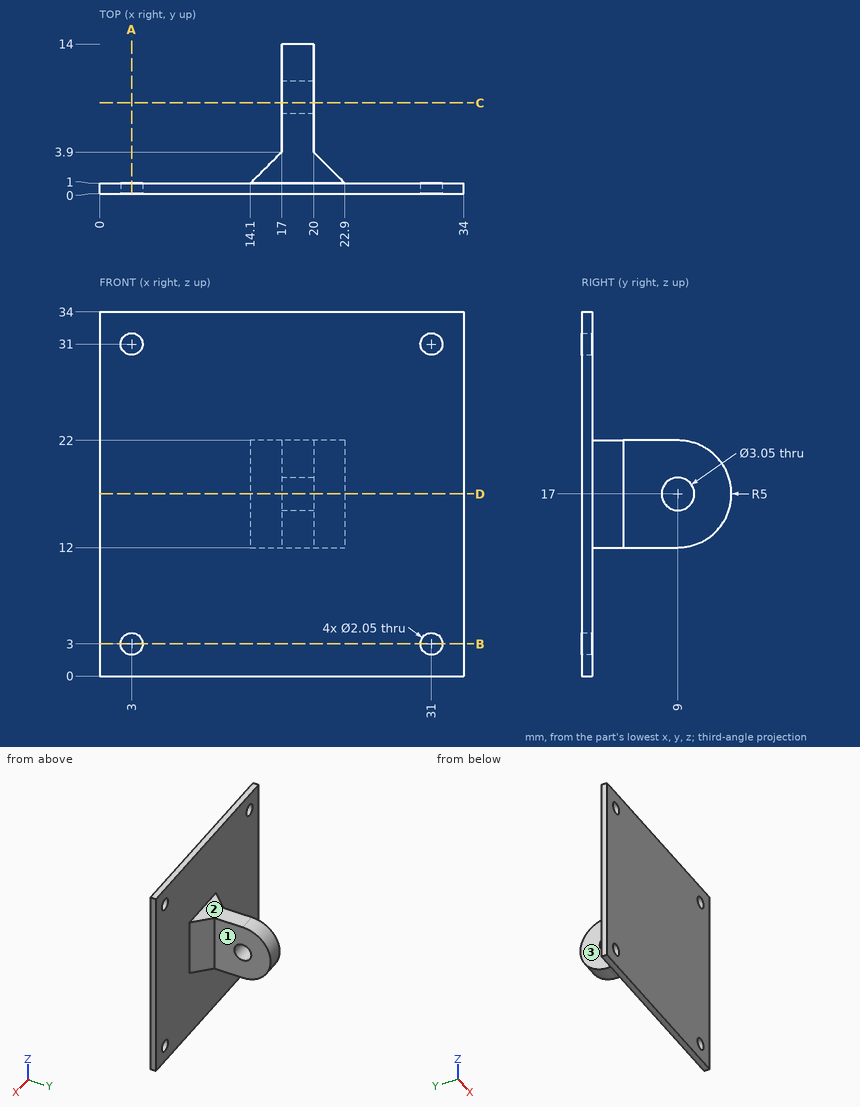
Job drawing, mm, ordinate dimensions from the low corner. One solid piece. A direction names the side the tool comes from. Coordinates: 2 decimals unless noted, no trailing zeros. Order: outer loops, then holes, each group sorted by start corner. A loop starts at its lowest first (then second) coordinate and runs counter-clockwise, first axis right, second up. Notation, with made-up numbers: (-25.5, 58.5) - (-4.5, 58.5) arc R25 cw to (-4.5, 84.5) - close; hole circle Ø5 at (61.5, -8). An arc over 180 degrees is marked (long way). Return JSON: item names as keys, results as strings. Group by question number.
1) Flat gauge pins, fed straight in: P1, Ø4, axis at y = 1.5, z = 19.5, coming from the +X side; P2, Ø2, axis at x = 26.5, z = 5, coming from the +Y side; P3, Ø3, axis at y = 11, z = 16, coming from the +X side; P4, Ø3, axis at y = 10, z = 18.5, coming from the -X side. Where does each tip first touch, or does it go through?
2) Saw through at B-B, the plane z = 3. Write the cut outline in (x, y) (3 decimals).
3) Saw through at D-D, the plane z = 17. Write the cut outline in (x, y) (3 decimals).
4) Saw through at C-C, the plane y = 8.5. Write the cut outline in (x, z), plus the area to 3 significant figures.
5) Probe line 1 (X direction, y = 0.5, z = 3) (3 decimals); line 2 (Y direction, x = 24, z = 10); line 3 (Y direction, x = 18, z = 17) (3 decimals). List the from-to ranges inside material, lowest first. Write a range as from..to.
6) Saw through at A-A, the plane x = 3. Write the cut outline in (y, z) (3 decimals), plus the area to 3 significant figures.
7) Tool access for the marked faces 1, 2 and 3: list every direction of +Z, -Z, +X, -X, +Y, -Y with a clear straight run to the whole face (end or side of a thin tool).
Values found:
{
 "1": {"P1": "stops at x = 34", "P2": "stops at y = 1", "P3": "stops at x = 20", "P4": "stops at x = 17"},
 "2": {"outline": "(0, 0) - (1.975, 0) - (1.975, 1) - (0, 1) - close; (4.025, 0) - (29.975, 0) - (29.975, 1) - (4.025, 1) - close; (32.025, 0) - (34, 0) - (34, 1) - (32.025, 1) - close"},
 "3": {"outline": "(0, 0) - (34, 0) - (34, 1) - (22.9, 1) - (20, 3.9) - (20, 7.475) - (17, 7.475) - (17, 3.9) - (14.1, 1) - (0, 1) - close; (17, 10.525) - (20, 10.525) - (20, 14) - (17, 14) - close"},
 "4": {"outline": "(17, 12) - (20, 12) - (20, 15.56) - (17, 15.56) - close; (17, 18.44) - (20, 18.44) - (20, 22) - (17, 22) - close", "area": "21.4 mm²"},
 "5": {"line 1": "x = 0..1.975, 4.025..29.975, 32.025..34", "line 2": "y = 0..1", "line 3": "y = 0..7.475, 10.525..14"},
 "6": {"outline": "(0, 0) - (1, 0) - (1, 1.975) - (0, 1.975) - close; (0, 4.025) - (1, 4.025) - (1, 29.975) - (0, 29.975) - close; (0, 32.025) - (1, 32.025) - (1, 34) - (0, 34) - close", "area": "29.9 mm²"},
 "7": {"face 1": "+Z, -Z, +X, +Y", "face 2": "+Z, +X, -X, +Y", "face 3": "+Z, -Z, -X, +Y"}
}
